from build123d import *

# Parameters (mm, degrees)
SKETCH1_R           = 2.75
BOSS_EXTRUDE1_DEPTH = 2


with BuildPart() as part:
    # Sketch1 → Boss-Extrude1 (new body, symmetric)
    with BuildSketch(Plane.XY):
        Polygon((-29, 0), (29, 0), (29, 18), (9, 58), (-9, 58), (-29, 18), align=None)
        with Locations((0, 9)):
            Circle(SKETCH1_R, mode=Mode.SUBTRACT)
        with Locations((-20, 9)):
            Circle(SKETCH1_R, mode=Mode.SUBTRACT)
        with Locations((20, 9)):
            Circle(SKETCH1_R, mode=Mode.SUBTRACT)
        with Locations((0, 29)):
            Circle(SKETCH1_R, mode=Mode.SUBTRACT)
        with Locations((0, 49)):
            Circle(SKETCH1_R, mode=Mode.SUBTRACT)
    extrude(amount=BOSS_EXTRUDE1_DEPTH, both=True)


solid = part.part
Work out the finished part from the listing and answer in its coordinate system (mm). Round coordinates to 2 decimals unless told otherwise and drop trailing zeros. Order: outer loops, then holes, each group sorted by start corner. A loop starts at its lowest first (then second) coordinate and runs counter-clockwise, first axis right, second up. Notation, with made-up numbers: M 4,33.5 L 23,33.5 A16 cw 23,57.5 Z; hole C -5.75,5.5 d2. An arc over 180 degrees is marked long. Put each result on its own line as item: value. Start each with the question number.
Q1. Straight lines are drawn through the part: L1, parallel to Y at x = 0, z = -0.2; L2, parallel to X at y = 8.5, z = -0.6; L3, parallel to Y at x = -20, z = 0.15. For each, find the intervals that lie inside material, in ascending order. Write a range as [from, to].
Q2. Section C-C, the plane x = 0 is taken. Write down the section's boundary in (y, z).
Q3. Section D-D, the plane y = 49 is taken. Write down the section's boundary in (x, z).
Q4. Section A-A, the plane y = 9 is taken. Write down the section's boundary in (x, z).
Q5. Flat-ended cylindrical pins translate along their axes: pin 1 (1 mm diameter, centred on y = 19.5, z = 0, fed in from +X); pin 2 (9 mm diameter, centred on x = 0, y = 49, fed in from +Z); pin 3 (1.5 mm diameter, centred on y = 48, z = -0.5, fed in from -X) (3 decimals); pin 4 (1.5 mm diameter, centred on y = 22.5, z = 1, fed in from -X) (3 decimals). Find the tip coordinate at first contact, or state that the pin passes through.
Q6. Section B-B, the plane x = 20 is taken. Write down the section's boundary in (y, z).
Q7. For a pull along Y with two mould halves and no side action, classify faces 1 (the cylindrical face through (-0.358, 51.727, -0.028)), 2 (the cylindrical face through (-0.358, 11.727, -0.028)), 3 (the flat face through (0, 0, 0)), 4 (the flat face through (19, 38, 0)) as pulls with the +Y half, pulls with the -Y half, needs draft (parallel to the pull), parting line crosses it, or undercut.
Findings below:
1. L1: y = [0, 6.25], [11.75, 26.25], [31.75, 46.25], [51.75, 58]
1. L2: x = [-29, -22.7], [-17.3, -2.7], [2.7, 17.3], [22.7, 29]
1. L3: y = [0, 6.25], [11.75, 36]
2. outline: M 0,-2 L 6.25,-2 L 6.25,2 L 0,2 Z; M 11.75,-2 L 26.25,-2 L 26.25,2 L 11.75,2 Z; M 31.75,-2 L 46.25,-2 L 46.25,2 L 31.75,2 Z; M 51.75,-2 L 58,-2 L 58,2 L 51.75,2 Z
3. outline: M -13.5,-2 L -2.75,-2 L -2.75,2 L -13.5,2 Z; M 2.75,-2 L 13.5,-2 L 13.5,2 L 2.75,2 Z
4. outline: M -29,-2 L -22.75,-2 L -22.75,2 L -29,2 Z; M -17.25,-2 L -2.75,-2 L -2.75,2 L -17.25,2 Z; M 2.75,-2 L 17.25,-2 L 17.25,2 L 2.75,2 Z; M 22.75,-2 L 29,-2 L 29,2 L 22.75,2 Z
5. pin 1: stops at x = 28.5
5. pin 2: stops at z = 2
5. pin 3: stops at x = -14.375
5. pin 4: stops at x = -27.125
6. outline: M 0,-2 L 6.25,-2 L 6.25,2 L 0,2 Z; M 11.75,-2 L 36,-2 L 36,2 L 11.75,2 Z
7. face 1: undercut
7. face 2: undercut
7. face 3: pulls with the -Y half
7. face 4: pulls with the +Y half
